```python
from build123d import *

# Parameters (mm, degrees)
F1_DEPTH  = 57.15
F2_R      = 6.35
F3_DEPTH  = 25.4
F3_FACE_R = 6.35
F4_DEPTH  = 25.401


with BuildPart() as f1:
    # F0 (on Front) → F1 (new body)
    with BuildSketch(Plane.XZ):
        Polygon((-127, 0), (0, 0), (0, 12.7), (-31.753481, 12.7), (-63.5, 12.7), (-95.243674, 12.7), (-127, 12.7), align=None)
        with BuildLine():
            Line((-63.5, 12.7), (-31.753481, 12.7))
            ThreePointArc((-31.753481, 12.7), (-40.651931, 16.338676), (-44.451393, 25.169669))
            ThreePointArc((-44.451393, 25.169669), (-44.453481, 25.4), (-44.451393, 25.630331))
            ThreePointArc((-44.451393, 25.630331), (-63.459927, 44.449958), (-82.54747, 25.71047))
            ThreePointArc((-82.54747, 25.71047), (-82.543674, 25.4), (-82.54747, 25.08953))
            ThreePointArc((-82.54747, 25.08953), (-86.373865, 16.310639), (-95.243674, 12.7))
            Line((-95.243674, 12.7), (-63.5, 12.7))
        make_face()
        with BuildLine():
            ThreePointArc((-50.8, 25.4), (-54.519744, 16.419744), (-63.5, 12.7))
            ThreePointArc((-63.5, 12.7), (-72.480256, 34.380256), (-50.8, 25.4))
        make_face(mode=Mode.SUBTRACT)
        with BuildLine():
            ThreePointArc((-44.451393, 25.630331), (-44.453481, 25.4), (-44.451393, 25.169669))
            ThreePointArc((-44.451393, 25.169669), (-44.45, 25.4), (-44.451393, 25.630331))
        make_face()
        with BuildLine():
            ThreePointArc((-82.54747, 25.71047), (-82.55, 25.4), (-82.54747, 25.08953))
            ThreePointArc((-82.54747, 25.08953), (-82.543674, 25.4), (-82.54747, 25.71047))
        make_face()
    extrude(amount=F1_DEPTH)

    # F2 (on Top) → F3 (join)
    with BuildSketch(Plane.XY):
        with Locations((-19.05, -28.575)):
            Circle(F2_R)
        with Locations((-107.95, -28.575)):
            Circle(F2_R)
    extrude(amount=F3_DEPTH)

    # F3_face (on face) → F4 (cut, through all)
    with BuildSketch(Plane(origin=(-107.95, -28.575, 25.4), x_dir=(1, 0, 0), z_dir=(0, 0, 1))):
        Circle(F3_FACE_R)
        with Locations((88.9, 0)):
            Circle(F3_FACE_R)
    extrude(amount=-F4_DEPTH, mode=Mode.SUBTRACT)


solid = f1.part
```
Model file for the job. Use its own axes, mm. A direction names the side the tool comes from. Coordinates: 2 decimals unless noted, no trailing zeros. Order: outer loops, then holes, each group sorted by start corner. A loop starts at its lowest first (then second) coordinate and runs counter-clockwise, first axis right, second up. Notation, with made-up numbers: M 78,80 L 128,80 A12 cw 128,92 Z; hole C -32.75,47.5 d10. An arc over 180 degrees is marked long. Answer as CSV lines item,"result".
(1) Band-saw the part on C-C, the plane z = 16.5. List the corners of the cut face in (x, y).
Geometry says:
outline,"M -86.18,-57.15 L -72.56,-57.15 L -72.56,0 L -86.18,0 Z; M -54.44,-57.15 L -40.81,-57.15 L -40.81,0 L -54.44,0 Z"
(2) Flat gauge pins, fed straight in: pin 1 (8 mm diameter, centred on y = -46, z = 32, fed in from -X); pin 2 (12 mm diameter, centred on y = -18.5, z = 35.5, fed in from -X); pin 3 (1.5 mm diameter, centred on y = -26.5, z = 23, fed in from -X). Where does each tip first touch, or does it go through?
Geometry says:
pin 1,"stops at x = -82.37"
pin 2,"stops at x = -82.1"
pin 3,"stops at x = -82.94"
(3) Pull direction Y, two halves, no side cores. Call faces 1 (the cylindrical face through (-112.63, -24.283, 6.439)), 2 (the cylindrical face through (-86.276, -28.175, 16.407)), 3 (the flat face through (-64, 0, 8)): +Y half, -Y half, draft (parallel to the pull), parting line (faces both ways), or undercut.
Geometry says:
face 1,"undercut"
face 2,"draft"
face 3,"+Y half"
(4) Band-saw the part on D-D, the plane z = 11. List the corners of the cut face in (x, y) (3 decimals), then the cut area to 3 significant figures.
Geometry says:
outline,"M -127,-57.15 L 0,-57.15 L 0,0 L -127,0 Z; hole C -107.95,-28.575 d12.7; hole C -19.05,-28.575 d12.7"
area,"7,000 mm2"
(5) 3-axis set-ups, long thin cutter, end or side, ignore diameter. For faces 4 (the flat face through (-111, -22, 12.7)), 5 (the flat face through (0, -28, 6)), 6 (the flat face through (-12, -28, 12.7)): which of +Z, -Z, +X, -X, +Y, -Y reach the whole face in a straight line?
Geometry says:
face 4,"+Z, -X, +Y, -Y"
face 5,"+Z, -Z, +X, +Y, -Y"
face 6,"+Z, +X, +Y, -Y"
(6) Wall check: line 1 along Y through (x, z) = (-19.05, 5.25) (3 decimals); line 2 along X through (y, z) = (-24, 25.4); line 3 along X through (y, z) = (-41, 25). Give the ranges that are in metal, low to high.
Geometry says:
line 1,"y = -57.15 to -34.925, -22.225 to 0"
line 2,"x = -82.55 to -76.2, -50.8 to -44.45"
line 3,"x = -82.55 to -76.19, -50.81 to -44.45"
(7) Band-saw the part on A-A, the plane x = -107.95. List the corners of the cut face in (y, z) (3 decimals), then the cut area to 3 significant figures.
Geometry says:
outline,"M -57.15,0 L -34.925,0 L -34.925,12.7 L -57.15,12.7 Z; M -22.225,0 L 0,0 L 0,12.7 L -22.225,12.7 Z"
area,"565 mm2"
(8) Band-saw the part on B-B, the plane y = -50. List the corners of the cut face in (x, z).
Geometry says:
outline,"M -127,0 L 0,0 L 0,12.7 L -31.75,12.7 A12.7 cw -44.45,25.17 A19.04 ccw -44.45,25.63 A19.05 ccw -82.55,25.71 A19.05 ccw -82.55,25.09 A12.7 cw -95.24,12.7 L -127,12.7 Z; hole C -63.5,25.4 d25.4"
